Read the model definition and answer for the solid it produces. Units are mm, in the model's axes. Coordinates: 2 decimals unless noted, no trailing zeros. Use a Markdown table: item, result. Add a question column.
1) Each of these flat-tipped pins is pushed along its axis until it touches: pin 1 Ø1 at (x, z) = (24.5, 13.5) entering from -Y; pin 2 Ø1 at (y, z) = (-123, 18) entering from -X; pin 3 Ø7.5 at (x, z) = (-66.675, 0) entering from -Y. Where does it stop, or does it pass through?
2) Find the intervals of material crossed by probe 1 along X at (y, z) = (-160.5, 0); probe 2 along X at (y, z) = (-144, 8.5); probe 3 along Z at (x, y) = (-10, 28.5), in increasing order. Write a range as [from, to].
3) The mould has two halves that part along X. Classify faces 1 (the face through (74.388, -53.355, -16.519)), 2 (the face through (-70.79, -199.8, -0.91)), 3 (the face through (56, 109.927, -45)): released by +X, released by -X, zero draft, split by the parting line, or undercut.
from build123d import *

# Parameters (mm, degrees)
CIRPATTERN1_COUNT              = 8
F_1_4_0_2500_DOWEL_HOLE1_D     = 6.35
F_1_4_0_2500_DOWEL_HOLE1_DEPTH = 9.906
F_1_4_0_2500_DOWEL_HOLE1_TIP   = 1.907732465


with BuildPart() as part:
    # Sketch1 → Revolve2 (revolve)
    with BuildSketch(Plane.XY, mode=Mode.PRIVATE) as revolve2_sk:
        with BuildLine():
            Line((71.638455479, 109.927347077), (76.2, 109.927347077))
            Line((76.2, 109.927347077), (76.2, -212.127673762))
            Line((76.2, -212.127673762), (53.792460107, -212.127673762))
            Line((53.792460107, -212.127673762), (53.792460107, -59.727673762))
            add(Edge.make_bspline(
                [(53.792460107, -59.727673762), (53.792458875, -59.657143693), (53.79192973, -59.515566639), (53.789553877, -59.181725153), (53.783229275, -58.904956029), (53.773743784, -58.532728024), (53.761100883, -58.212998158), (53.741350051, -57.781754979), (53.711337705, -57.281120436), (53.667125535, -56.688158703), (53.588220857, -55.848640904), (53.488359258, -55.0083264), (53.367608174, -54.172595971), (53.197743199, -53.172585782), (53.002996554, -52.177603366), (52.777307477, -51.18869963), (52.520946571, -50.207649587), (52.240221677, -49.233238292), (51.935281065, -48.266129779), (51.544470146, -47.149295627), (51.050452662, -45.89056897), (50.509666041, -44.651129374), (49.922993204, -43.432862102), (49.291052494, -42.237253822), (48.61505748, -41.066315469), (47.895407759, -39.921133254), (47.134034366, -38.804236844), (46.430801278, -37.851612398), (45.804470147, -37.055832742), (45.263749884, -36.403541907), (44.826059146, -35.894408262), (44.425708383, -35.447153291), (44.092389692, -35.084791822), (43.78485681, -34.760500791), (43.58500459, -34.551710093), (43.355324254, -34.318676932), (43.254715332, -34.217322701), (43.204843184, -34.167450314)],
                knots=[0.082637729, 0.082637729, 0.082637729, 0.082637729, 0.082637729, 0.092574926, 0.102512123, 0.11244932, 0.122386517, 0.132323714, 0.142260911, 0.162135305, 0.182009699, 0.201884093, 0.24163288, 0.261507274, 0.281381668, 0.321130456, 0.360879243, 0.380753637, 0.400628031, 0.440376819, 0.480125606, 0.519874394, 0.559623181, 0.599371969, 0.639120757, 0.678869544, 0.718618332, 0.75836712, 0.798115907, 0.817990301, 0.837864695, 0.857739089, 0.877613483, 0.88755068, 0.897487877, 0.907425074, 0.91736227, 0.91736227, 0.91736227, 0.91736227, 0.91736227], degree=4))
            Line((43.204843184, -34.167450314), (34.597214986, -25.559822117))
            add(Edge.make_bspline(
                [(24.01, 0), (24.010001231, -0.070528647), (24.010530378, -0.21358419), (24.012906064, -0.543182916), (24.019230459, -0.824160397), (24.02871558, -1.194822071), (24.041357874, -1.513435058), (24.057158098, -1.861939603), (24.076113357, -2.193706871), (24.103750972, -2.6180694), (24.14321918, -3.122033947), (24.214231842, -3.879978675), (24.334058815, -4.886450388), (24.510418183, -6.05671076), (24.761817375, -7.385166415), (25.062727459, -8.703574514), (25.412702772, -10.009637209), (25.811293135, -11.301819597), (26.257877546, -12.578099335), (26.75193548, -13.836887484), (27.292605281, -15.076197129), (27.879411549, -16.294609794), (28.511071563, -17.489938794), (29.187464564, -18.661287757), (29.906377272, -19.805743397), (30.668954172, -20.923860075), (31.370099368, -21.87441176), (31.9996683, -22.673445481), (32.535060595, -23.320422138), (32.983187947, -23.840005017), (33.419382207, -24.329816247), (33.846758303, -24.78848439), (34.156490822, -25.113868311), (34.44779214, -25.409649047), (34.547344609, -25.509949933), (34.597214986, -25.559822117)],
                knots=[0.082637729, 0.082637729, 0.082637729, 0.082637729, 0.082637729, 0.092574926, 0.102512123, 0.11244932, 0.122386517, 0.132323714, 0.142260911, 0.152198108, 0.162135305, 0.182009699, 0.201884093, 0.24163288, 0.281381668, 0.321130456, 0.360879243, 0.400628031, 0.440376819, 0.480125606, 0.519874394, 0.559623181, 0.599371969, 0.639120757, 0.678869544, 0.718618332, 0.75836712, 0.798115907, 0.817990301, 0.837864695, 0.857739089, 0.877613483, 0.897487877, 0.907425074, 0.91736227, 0.91736227, 0.91736227, 0.91736227, 0.91736227], degree=4))
            add(Edge.make_bspline(
                [(24.01, 0), (24.010000626, 0.035892652), (24.010538457, 0.11011369), (24.012955849, 0.267641069), (24.019393694, 0.427064117), (24.031465725, 0.646764266), (24.052367213, 0.901433328), (24.086116845, 1.202537273), (24.137431431, 1.542050498), (24.201475827, 1.880996777), (24.278073727, 2.21635442), (24.367255697, 2.549239421), (24.468673539, 2.878092645), (24.582551197, 3.203347041), (24.708128897, 3.523627157), (24.846218103, 3.839666733), (24.995002427, 4.149282184), (25.156944348, 4.454783123), (25.327420631, 4.751301575), (25.513446847, 5.045703861), (25.702720396, 5.325518936), (25.9153376, 5.610727543), (26.0898085, 5.832913647), (26.277277882, 6.049951637), (26.415487374, 6.208641646), (26.581374196, 6.382121779), (26.655452387, 6.458478841), (26.706211329, 6.50923965)],
                knots=[0.082568816, 0.082568816, 0.082568816, 0.082568816, 0.082568816, 0.102426634, 0.122284453, 0.142142271, 0.162000089, 0.201715725, 0.241431362, 0.281146998, 0.320862634, 0.360578271, 0.400293907, 0.440009544, 0.47972518, 0.519440816, 0.559156453, 0.598872089, 0.638587725, 0.678303362, 0.718018998, 0.757734635, 0.797450271, 0.837165907, 0.857023726, 0.876881544, 0.91659718, 0.91659718, 0.91659718, 0.91659718, 0.91659718], degree=4))
            add(Edge.make_bspline(
                [(26.706211329, 6.50923965), (49.172333461, 34.635954224), (71.638455479, 109.927347077)],
                knots=[0, 0, 0, 1, 1, 1], degree=2))
        make_face()
    revolve(revolve2_sk.sketch.rotate(Axis((0, 0, 0), (0, -1, 0)), 90), axis=Axis((0, 0, 0), (0, -1, 0)))

    # Sketch4 → 3/8-24 Tapped Hole1 (revolve, cut)
    with BuildSketch(Plane(origin=(66.675, -212.127673762, 0), x_dir=(0, 0, -1), z_dir=(1, 0, 0))):
        Polygon((0, 0), (0, 27.534688714), (4.2164, 25.00122), (4.2164, 0), align=None)
    f_3_8_24_tapped_hole1 = revolve(axis=Axis((66.675, -218.477673762, 0), (0, 1, 0)), mode=Mode.SUBTRACT)

    # CirPattern1: 3/8-24 Tapped Hole1 ×8 about axis
    cirpattern1_axis = Axis((0, 0, 0), (0, 1, 0))
    for i in range(1, CIRPATTERN1_COUNT):
        add(f_3_8_24_tapped_hole1.rotate(cirpattern1_axis, i * 360 / CIRPATTERN1_COUNT), mode=Mode.SUBTRACT)

    # 1/4 (0.2500) Dowel Hole1
    with Locations(Plane(origin=(0, -212.127673762, 0), x_dir=(-1, 0, 0), z_dir=(0, -1, 0))):
        with Locations((-61.59966783, 25.515417853), (61.59966783, -25.515417853)):
            Hole(F_1_4_0_2500_DOWEL_HOLE1_D / 2, depth=F_1_4_0_2500_DOWEL_HOLE1_DEPTH)
            with Locations((0, 0, -(F_1_4_0_2500_DOWEL_HOLE1_DEPTH + F_1_4_0_2500_DOWEL_HOLE1_TIP / 2))):  # 118° drill point
                Cone(0, F_1_4_0_2500_DOWEL_HOLE1_D / 2, F_1_4_0_2500_DOWEL_HOLE1_TIP, mode=Mode.SUBTRACT)


solid = part.part
Check result:
| question | item | result |
|---|---|---|
| 1 | pin 1 | stops at y = -17.4 |
| 1 | pin 2 | stops at x = -74.16 |
| 1 | pin 3 | stops at y = -186.85 |
| 2 | probe 1 | x = [-76.2, -53.79], [53.79, 76.2] |
| 2 | probe 2 | x = [-75.72, -53.12], [53.12, 75.72] |
| 2 | probe 3 | z = [-75.54, -39.4], [39.4, 75.54] |
| 3 | face 1 | split by the parting line |
| 3 | face 2 | undercut |
| 3 | face 3 | zero draft |
